from build123d import *

# Parameters (mm, degrees)
SKETCH1_R           = 6.5
BOSS_EXTRUDE1_DEPTH = 10
SKETCH2_R           = 5
BOSS_EXTRUDE2_DEPTH = 30
CUT_EXTRUDE1_DEPTH  = 9


with BuildPart() as part:
    # Sketch1 → Boss-Extrude1 (new body)
    with BuildSketch(Plane.XY):
        Circle(SKETCH1_R)
    extrude(amount=-BOSS_EXTRUDE1_DEPTH)

    # Sketch2 → Boss-Extrude2 (add)
    with BuildSketch(Plane(origin=(0, 0, -10), x_dir=(-1, 0, 0), z_dir=(0, 0, -1))):
        Circle(SKETCH2_R)
    extrude(amount=BOSS_EXTRUDE2_DEPTH)

    # Sketch3 → Cut-Extrude1 (cut)
    with BuildSketch(Plane.XY):
        Polygon((-2.552781944, 4.525848467), (-5.195890718, 0.052150219), (-2.643108774, -4.473698247), (2.552781944, -4.525848467), (5.195890718, -0.052150219), (2.643108774, 4.473698247), align=None)
    extrude(amount=-CUT_EXTRUDE1_DEPTH, mode=Mode.SUBTRACT)


solid = part.part
For this review, take the finished solid that the model builds, in its own axes (mm). A direction names the side the tool comes from. Coordinates: 2 decimals unless noted, no trailing zeros. Write each loop counter-clockwise with the first axis right and the second up, starting at its lowest first coordinate (ties: lowest second). Pieces come first, ordered by that corner, then holes. Notation, with made-up numbers: (36, -18.5) -> (57, -18.5) arc R14 cw to (57, -14.5) -> close; hole circle Ø9 at (-22, -19.5). An arc over 180 degrees is marked (long way). Write each question's results on one line, items separated by ' | '. Start each with the question number.
1) Consider section B-B (y = 2.25). Write out the cut boundary in (x, z), plus the area to 3 significant figures.
2) Consider section A-A (z = -4). Write out the cut boundary in (x, y).
3) Wall thickness on L1, parallel to Z at x = -5.25, y = -3.25; L2, parallel to Z at x = 4, y = 0.5; L3, parallel to Y at x = 2, z = -4: over which ranges is each line inside the solid? List them lowest first. Write a range as [from, to].
4) Consider section D-D (z = -17). Write out the cut boundary in (x, y).
5) Consider section C-C (x = 0.75). Write out the cut boundary in (y, z), plus the area to 3 significant figures.
6) For faces 4 (the face through (1.08, -4.88, -24.79)), 5 (the face through (4, -3, 0)), 6 (the face through (3.856, -2.32, -4.437)), list the 3-axis set-ups (+Z, -Z, +X, -X, +Y, -Y) from which the entire face can be reached by the end or side of a thin tool; tool diameter is ignored.
7) Insertion check: pin 1 (1.5 mm diameter, centred on x = -3, z = -26, fed in from -Y); pin 2 (6 mm diameter, centred on y = -5, z = -23.5, fed in from -X). Each pin has a flat end and moves straight along its axis. Give the tip position at first contact, or say it passes through.
8) The part is to be moulded in two halves that separate along X. For faces 1 (the face through (-5.158, -3.955, -4.93)), 2 (the face through (0, 0, -40)), 3 (the face through (0, 0, -9)), say which applies: +X half, -X half, draft (parallel to the pull), parting line (faces both ways), or undercut.
Geometry says:
1) outline: (-6.1, -10) -> (-4.47, -10) -> (-4.47, -40) -> (4.47, -40) -> (4.47, -10) -> (6.1, -10) -> (6.1, 0) -> (3.9, 0) -> (3.9, -9) -> (-3.9, -9) -> (-3.9, 0) -> (-6.1, 0) -> close | area: 320 mm^2
2) outline: circle Ø13 at (0, 0); hole (-5.2, 0.05) -> (-2.64, -4.47) -> (2.55, -4.53) -> (5.2, -0.05) -> (2.64, 4.47) -> (-2.55, 4.53) -> close
3) L1: [-10, 0] | L2: [-40, -9] | L3: [-6.18, -4.52], [4.48, 6.18]
4) outline: circle Ø10 at (0, 0)
5) outline: (-6.46, -10) -> (-4.94, -10) -> (-4.94, -40) -> (4.94, -40) -> (4.94, -10) -> (6.46, -10) -> (6.46, 0) -> (4.49, 0) -> (4.49, -9) -> (-4.51, -9) -> (-4.51, 0) -> (-6.46, 0) -> close | area: 345 mm^2
6) face 4: -Z | face 5: +Z, +X, -X, +Y, -Y | face 6: +Z
7) pin 1: y = -4.47 | pin 2: x = -4.58
8) face 1: parting line | face 2: draft | face 3: undercut
